```python
from build123d import *

# Parameters (mm, degrees)
BOSS_EXTRUDE1_DEPTH = 5
SKETCH2_R           = 1.25
CUT_EXTRUDE1_DEPTH  = 10
SKETCH3_R           = 10
CUT_EXTRUDE2_DEPTH  = 116
CIRPATTERN1_COUNT   = 3


with BuildPart() as part:
    # Sketch1 → Boss-Extrude1 (new, symmetric)
    with BuildSketch(Plane.XY):
        Polygon((-43.301270189, -75), (43.301270189, -75), (86.602540378, 0), (43.301270189, 75), (-43.301270189, 75), (-86.602540378, 0), align=None)
    extrude(amount=BOSS_EXTRUDE1_DEPTH, both=True)

    # Sketch2 → Cut-Extrude1 (cut)
    with BuildSketch(Plane.XZ.offset(75)):
        with Locations(Location((-33.301270189, 0, 0), (0, 0, 270))):
            Circle(SKETCH2_R)
        with Locations(Location((-23.301270189, 0, 0), (0, 0, 270))):
            Circle(SKETCH2_R)
        with Locations(Location((23.301270189, 0, 0), (0, 0, 90))):
            Circle(SKETCH2_R)
        with Locations(Location((33.301270189, 0, 0), (0, 0, 90))):
            Circle(SKETCH2_R)
    cut_extrude1 = extrude(amount=-CUT_EXTRUDE1_DEPTH, mode=Mode.SUBTRACT)

    # Sketch3 → Cut-Extrude2 (cut, through all)
    with BuildSketch(Plane.XY.offset(5)):
        Circle(SKETCH3_R)
    extrude(amount=-CUT_EXTRUDE2_DEPTH, mode=Mode.SUBTRACT)

    # CirPattern1: Cut-Extrude1 ×3 about axis
    cirpattern1_axis = Axis((0, 0, 0), (0, 0, 1))
    for i in range(1, CIRPATTERN1_COUNT):
        add(cut_extrude1.rotate(cirpattern1_axis, i * 360 / CIRPATTERN1_COUNT), mode=Mode.SUBTRACT)


solid = part.part
```
Model file for the job. Use its own axes, mm. Round coordinates to 2 decimals unless told otherwise and drop trailing zeros. Order: outer loops, then holes, each group sorted by start corner. A loop starts at its lowest first (then second) coordinate and runs counter-clockwise, first axis right, second up. Notation, with made-up numbers: (40, 38.25) -> (77, 38.25) arc R17 cw to (77, 57.25) -> close; hole circle Ø8 at (77, -39.75). An arc over 180 degrees is marked (long way). Use one line per item in the form item = value.
Item 1: Cut at A-A, the plane x = 0. Write the cut outline in (y, z), and give its area (3 significant figures).
Returned:
outline = (-75, -5) -> (-10, -5) -> (-10, 5) -> (-75, 5) -> close; (10, -5) -> (75, -5) -> (75, 5) -> (10, 5) -> close
area = 1,300 mm^2
Item 2: Cut at D-D, the plane x = 59. Write the cut outline in (y, z), and give its area (3 significant figures).
Returned:
outline = (-47.81, -5) -> (47.81, -5) -> (47.81, 5) -> (-47.81, 5) -> close
area = 956 mm^2
Item 3: Flat gauge pins, fed straight in: pin 1 Ø2 at (x, z) = (-23.3, 0) entering from -Y; pin 2 Ø0.8 at (x, z) = (-32.5, 0.5) entering from -Y; pin 3 Ø18 at (x, y) = (0, 0) entering from -Z; pin 4 Ø1 at (y, z) = (43, -0.5) entering from +X. Where does each tip first touch, or does it go through?
Returned:
pin_1 = -65
pin_2 = -75
pin_3 = through
pin_4 = 62.07
Item 4: Drill centre lines: line 1 (X direction, y = -72.5, z = 0); line 2 (X direction, y = -67, z = 0); line 3 (X direction, y = 62.5, z = -0.25). Where is each one in solid material? Low to high.
Returned:
line_1 = -44.74 to -34.55, -32.05 to -24.55, -22.05 to 22.05, 24.55 to 32.05, 34.55 to 44.74
line_2 = -47.92 to -34.55, -32.05 to -24.55, -22.05 to 22.05, 24.55 to 32.05, 34.55 to 47.92
line_3 = -50.52 to -44.1, -39.2 to 39.2, 44.1 to 50.52
Item 5: Cut at B-B, the plane z = -3.5. Write the cut outline in (x, y), and give its area (3 significant figures).
Returned:
outline = (-86.6, 0) -> (-43.3, -75) -> (43.3, -75) -> (86.6, 0) -> (43.3, 75) -> (-43.3, 75) -> close; hole circle Ø20 at (0, 0)
area = 19,200 mm^2
Item 6: Pull direction X, two halves, no side cores. Call faces 1 (the face through (-65.255, -36.975, 0.07)), 2 (the face through (77.888, 5.235, -0.577)), 3 (the face through (1, 75, 0)): released by +X, released by -X, zero draft, split by the parting line, or undercut.
Returned:
face_1 = released by -X
face_2 = undercut
face_3 = zero draft
Item 7: Cut at C-C, the plane y = -60. Write the cut outline in (x, z).
Returned:
outline = (-51.96, -5) -> (51.96, -5) -> (51.96, 5) -> (-51.96, 5) -> close
